Read the model definition and answer for the solid it produces. Units are mm, in the model's axes. Give positions to 0.01 mm unless a question says otherwise; leave off trailing zeros. Loops run counter-clockwise (first coordinate to the right, second up) from the corner with the lowest first, then second, coordinate; pieces in that order, holes last.
(1) Straight lines are drawn through the part: probe 1 along Z at (x, y) = (3, -8); probe 2 along Z at (x, y) = (-552, -7); probe 3 along X at (y, z) = (-12.5, 220). For each, find the intervals that lie inside material, in ascending order.
(2) Each of these flat-tipped pins is pushed along its axis until it touches: P1, Ø2, axis at x = 422.5, y = -23.5, coming from the +Z side; P2, Ø3, axis at x = 381, y = -5, coming from the +Z side; P3, Ø16, axis at x = 464.79, z = -402.74, coming from the -Y side. Where does it stop, or does it pass through?
(3) Find section A-A, the plane y = -12.5. Write down the section's boundary in (x, z), then the cut area to 3 significant figures.
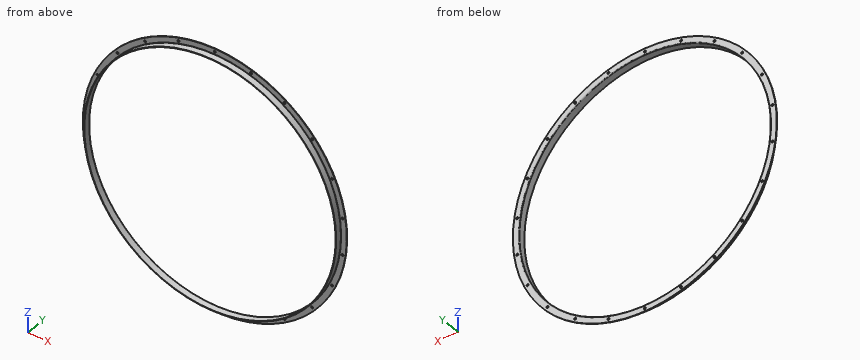
```python
from build123d import *

# Parameters (mm, degrees)
SKETCH1_R          = 630
SKETCH1_R_2        = 600
BASE_FLANGE1_DEPTH = 2.5
SKETCH8_R          = 5
CUT_EXTRUDE1_DEPTH = 10


# Read off the part's stored shape, not the designer's step: Edge-Flange1
# Sheet-metal steps are written as plain solids
with BuildPart() as part:
    # Sketch1 → Base-Flange1 (new body)
    with BuildSketch(Plane(origin=(0, 0, 0), x_dir=(1, 0, 0), z_dir=(0, 1, 0))):
        with Locations(Location((0, 0, 0), (0, 0, 270))):
            Circle(SKETCH1_R)
        with Locations(Location((0, 0, 0), (0, 0, 270))):
            Circle(SKETCH1_R_2, mode=Mode.SUBTRACT)
    extrude(amount=-BASE_FLANGE1_DEPTH)

    # Edge-Flange1 outline → Edge-Flange1 (revolve, cut)
    with BuildSketch(Plane.XY):
        with BuildLine():
            Line((600, -2.5), (600.145898034, -2.5))
            ThreePointArc((600.145898034, -2.5), (601.408349934, -0.69375696), (603.5, 0))
            Line((603.5, 0), (600, 0))
            Line((600, 0), (600, -2.5))
        make_face()
    revolve(axis=Axis((0, 0, 0), (0, 1, 0)), mode=Mode.SUBTRACT)

    # Edge-Flange1 2 outline → Edge-Flange1 2 (revolve)
    with BuildSketch(Plane.XY):
        with BuildLine():
            Line((600, -3.5), (600, -33.5))
            Line((600, -33.5), (602.5, -33.5))
            Line((602.5, -33.5), (602.5, -3.5))
            ThreePointArc((602.5, -3.5), (602.792893219, -2.792893219), (603.5, -2.5))
            Line((603.5, -2.5), (600.145898034, -2.5))
            ThreePointArc((600.145898034, -2.5), (600.036666571, -2.994706462), (600, -3.5))
        make_face()
    revolve(axis=Axis((0, 0, 0), (0, 1, 0)))

    # Sketch8 → Cut-Extrude1 (cut)
    with BuildSketch(Plane(origin=(0, 0, 0), x_dir=(1, 0, 0), z_dir=(0, 1, 0))):
        with Locations(Location((173.265522457, 590.088178773, 0), (0, 0, 270))):
            Circle(SKETCH8_R)
        with Locations(Location((332.494102735, 517.370922691, 0), (0, 0, 270))):
            Circle(SKETCH8_R)
        with Locations(Location((0, 615, 0), (0, 0, 270))):
            Circle(SKETCH8_R)
        with Locations(Location((464.785988228, 402.739351376, 0), (0, 0, 270))):
            Circle(SKETCH8_R)
        with Locations(Location((559.423677143, 255.480232996, 0), (0, 0, 270))):
            Circle(SKETCH8_R)
        with Locations(Location((608.740186757, 87.523625538, 0), (0, 0, 270))):
            Circle(SKETCH8_R)
        with Locations(Location((608.740186757, -87.523625538, 0), (0, 0, 270))):
            Circle(SKETCH8_R)
        with Locations(Location((559.423677143, -255.480232996, 0), (0, 0, 270))):
            Circle(SKETCH8_R)
        with Locations(Location((464.785988228, -402.739351376, 0), (0, 0, 270))):
            Circle(SKETCH8_R)
        with Locations(Location((332.494102735, -517.370922691, 0), (0, 0, 270))):
            Circle(SKETCH8_R)
        with Locations(Location((173.265522458, -590.088178773, 0), (0, 0, 270))):
            Circle(SKETCH8_R)
        with Locations(Location((0, -615, 0), (0, 0, 270))):
            Circle(SKETCH8_R)
        with Locations(Location((-173.265522457, -590.088178773, 0), (0, 0, 270))):
            Circle(SKETCH8_R)
        with Locations(Location((-332.494102735, -517.370922691, 0), (0, 0, 270))):
            Circle(SKETCH8_R)
        with Locations(Location((-464.785988228, -402.739351376, 0), (0, 0, 270))):
            Circle(SKETCH8_R)
        with Locations(Location((-559.423677143, -255.480232996, 0), (0, 0, 270))):
            Circle(SKETCH8_R)
        with Locations(Location((-608.740186757, -87.523625538, 0), (0, 0, 270))):
            Circle(SKETCH8_R)
        with Locations(Location((-608.740186757, 87.523625538, 0), (0, 0, 270))):
            Circle(SKETCH8_R)
        with Locations(Location((-559.423677143, 255.480232996, 0), (0, 0, 270))):
            Circle(SKETCH8_R)
        with Locations(Location((-464.785988228, 402.739351376, 0), (0, 0, 270))):
            Circle(SKETCH8_R)
        with Locations(Location((-332.494102735, 517.370922691, 0), (0, 0, 270))):
            Circle(SKETCH8_R)
        with Locations(Location((-173.265522457, 590.088178773, 0), (0, 0, 270))):
            Circle(SKETCH8_R)
    extrude(amount=-CUT_EXTRUDE1_DEPTH, mode=Mode.SUBTRACT)


solid = part.part
```
Entries:
1. probe 1: z = -602.49 to -599.99, 599.99 to 602.49
1. probe 2: z = -241.46 to -235.15, 235.15 to 241.46
1. probe 3: x = -560.9 to -558.21, 558.21 to 560.9
2. P1: stops at z = 430.52
2. P2: stops at z = 467.96
2. P3: stops at y = -2.5
3. outline: circle Ø1205 at (0, 0); hole circle Ø1200 at (0, 0)
3. area: 9,440 mm2
